Read the model definition and answer for the solid it produces. Units are mm, in the model's axes. Give positions to 0.01 mm unless a question says otherwise; leave off trailing zeros. Order: outer loops, then holes, each group sorted by start corner. A loop starts at its lowest first (then second) coordinate and runs counter-clockwise, first axis right, second up.
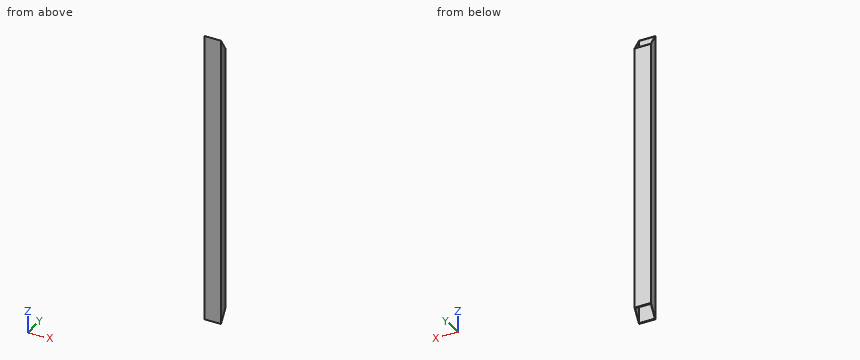
```python
from build123d import *

# Parameters (mm, degrees)
BOSS_EXTRUDE1_DEPTH = 700
SKETCH4_W           = 38
SKETCH4_H           = 18
CUT_EXTRUDE2_DEPTH  = 701
CUT_EXTRUDE1_DEPTH  = 41


with BuildPart() as part:
    # Sketch1 → Boss-Extrude1 (new body)
    with BuildSketch(Plane.XY):
        Polygon((20, -8), (0, -8), (-20, -8), (-20, 12), (20, 12), align=None)
    extrude(amount=BOSS_EXTRUDE1_DEPTH)

    # Sketch4 → Cut-Extrude2 (cut, through all)
    with BuildSketch(Plane.XY.offset(700)):
        with Locations((0, 2)):
            Rectangle(SKETCH4_W, SKETCH4_H)
    extrude(amount=-CUT_EXTRUDE2_DEPTH, mode=Mode.SUBTRACT)

    # Sketch3 → Cut-Extrude1 (cut, through all)
    with BuildSketch(Plane.ZY.offset(20)):
        Polygon((0, 12), (30, 12), (0, -8), align=None)
        Polygon((670, 12), (700, 12), (700, -8), align=None)
    extrude(amount=-CUT_EXTRUDE1_DEPTH, mode=Mode.SUBTRACT)


solid = part.part
```
1) The part is cut by section B-B on z = 115.5. Determine the outline of the cut face in (x, y).
Final values:
outline: (-20, -8) - (20, -8) - (20, 12) - (-20, 12) - close; hole (-19, -7) - (19, -7) - (19, 11) - (-19, 11) - close
2) Given pin 1 (5 mm diameter, centred on x = 13, y = 6.5, fed in from -Z), flat-ended and moving along its own axis, determine where the tip first touches the part or whether it passes through.
Final values:
pin 1: passes through
3) The part is cut by section C-C on x = -10. Determine the outline of the cut face in (y, z), and give its area (3 significant figures).
Final values:
outline: (-8, 0) - (-7, 1.5) - (-7, 698.5) - (-8, 700) - close; (11, 28.5) - (12, 30) - (12, 670) - (11, 671.5) - close
area: 1,340 mm2
4) Consider L1, parallel to Y at x = 10, z = 666; L2, parallel to X at y = -3.5, z = 205. Determine where each line is inside the solid, lowest interval first.
Final values:
L1: y = -8 to -7, 11 to 12
L2: x = -20 to -19, 19 to 20
5) The part is cut by section A-A on y = 4. Determine the outline of the cut face in (x, z).
Final values:
outline: (-20, 18) - (-19, 18) - (-19, 682) - (-20, 682) - close; (19, 18) - (20, 18) - (20, 682) - (19, 682) - close
